from build123d import *

# Parameters (mm, degrees)
EXTRUDE_1_DEPTH     = 5
EXTRUDE_1_2_DEPTH   = 5
EXTRUDE_1_3_DEPTH   = 5
EXTRUDE_1_4_DEPTH   = 5
EXTRUDE_3_DEPTH     = 2
SKETCH_3_W          = 20
SKETCH_3_H          = 19.604409946
CUT_EXTRUDE_1_DEPTH = 2
SKETCH_4_R          = 1.5
CUT_EXTRUDE_2_DEPTH = 12
SKETCH_6_W          = 24.27884079
SKETCH_6_H          = 14.237664084
CUT_EXTRUDE_5_DEPTH = 10


with BuildPart() as part:
    # Sketch 1 → Extrude 1 (new body)
    with BuildSketch(Plane.XY):
        with BuildLine():
            Line((13.964240044, 24), (-13.964240044, 24))
            ThreePointArc((-13.964240044, 24), (0, 11), (13.964240044, 24))
        make_face()
    extrude(amount=-EXTRUDE_1_DEPTH)



with BuildPart() as body_2:
    # Sketch 1 → Extrude 1 2 (new body)
    with BuildSketch(Plane.XY):
        with BuildLine():
            ThreePointArc((-18, -12.124355653), (-11, 0), (-18, 12.124355653))
            Line((-18, 12.124355653), (-18, -12.124355653))
        make_face()
    extrude(amount=-EXTRUDE_1_2_DEPTH)


with BuildPart() as body_3:
    # Sketch 1 → Extrude 1 3 (new body)
    with BuildSketch(Plane.XY):
        with BuildLine():
            Line((18, -12.124355653), (18, 12.124355653))
            ThreePointArc((18, 12.124355653), (11, 0), (18, -12.124355653))
        make_face()
    extrude(amount=-EXTRUDE_1_3_DEPTH)


with BuildPart() as body_4:
    # Sketch 1 → Extrude 1 4 (new body)
    with BuildSketch(Plane.XY):
        with BuildLine():
            ThreePointArc((13.964240044, -24), (0, -11), (-13.964240044, -24))
            Line((-13.964240044, -24), (13.964240044, -24))
        make_face()
    extrude(amount=-EXTRUDE_1_4_DEPTH)


with BuildPart() as part_1:
    add(part.part)

    add(body_2.part)  # Extrude 3 merges body 2

    add(body_3.part)  # Extrude 3 merges body 3

    add(body_4.part)  # Extrude 3 merges body 4
    # Sketch 2 → Extrude 3 (add)
    with BuildSketch(Plane.XY):
        with BuildLine():
            ThreePointArc((-18, 22.45), (-19.096015511, 25.096015511), (-16.45, 24))
            Line((-16.45, 24), (-12.139420395, 24))
            ThreePointArc((-12.139420395, 24), (-22.14405558, 28.14405558), (-18, 18.139420395))
            Line((-18, 18.139420395), (-18, 22.45))
        make_face()
        with BuildLine():
            Line((-12.139420395, 24), (-16.45, 24))
            ThreePointArc((-16.45, 24), (-16.903984489, 22.903984489), (-18, 22.45))
            Line((-18, 22.45), (-18, 18.139420395))
            ThreePointArc((-18, 18.139420395), (-13.85594442, 19.85594442), (-12.139420395, 24))
        make_face()
        with BuildLine():
            Line((12.139420395, 24), (-12.139420395, 24))
            ThreePointArc((-12.139420395, 24), (-13.85594442, 19.85594442), (-18, 18.139420395))
            Line((-18, 18.139420395), (-18, 12.124355653))
            ThreePointArc((-18, 12.124355653), (-11, 0), (-18, -12.124355653))
            Line((-18, -12.124355653), (-18, -18.139420395))
            ThreePointArc((-18, -18.139420395), (-13.85594442, -19.85594442), (-12.139420395, -24))
            Line((-12.139420395, -24), (12.139420395, -24))
            ThreePointArc((12.139420395, -24), (13.85594442, -19.85594442), (18, -18.139420395))
            Line((18, -18.139420395), (18, 18.139420395))
            ThreePointArc((18, 18.139420395), (13.85594442, 19.85594442), (12.139420395, 24))
        make_face()
        with BuildLine():
            ThreePointArc((-18, -12.124355653), (-11, 0), (-18, 12.124355653))
            Line((-18, 12.124355653), (-18, -12.124355653))
        make_face()
        with BuildLine():
            ThreePointArc((23.860579605, 24), (18, 29.860579605), (12.139420395, 24))
            Line((12.139420395, 24), (16.45, 24))
            ThreePointArc((16.45, 24), (18, 25.55), (19.55, 24))
            ThreePointArc((19.55, 24), (19.096015511, 22.903984489), (18, 22.45))
            Line((18, 22.45), (18, 18.139420395))
            ThreePointArc((18, 18.139420395), (22.14405558, 19.85594442), (23.860579605, 24))
        make_face()
        with BuildLine():
            Line((16.45, 24), (12.139420395, 24))
            ThreePointArc((12.139420395, 24), (13.85594442, 19.85594442), (18, 18.139420395))
            Line((18, 18.139420395), (18, 22.45))
            ThreePointArc((18, 22.45), (16.903984489, 22.903984489), (16.45, 24))
        make_face()
        with BuildLine():
            ThreePointArc((-12.139420395, -24), (-13.85594442, -19.85594442), (-18, -18.139420395))
            Line((-18, -18.139420395), (-18, -22.45))
            ThreePointArc((-18, -22.45), (-16.903984489, -22.903984489), (-16.45, -24))
            Line((-16.45, -24), (-12.139420395, -24))
        make_face()
        with BuildLine():
            Line((-18, -22.45), (-18, -18.139420395))
            ThreePointArc((-18, -18.139420395), (-22.14405558, -28.14405558), (-12.139420395, -24))
            Line((-12.139420395, -24), (-16.45, -24))
            ThreePointArc((-16.45, -24), (-19.096015511, -25.096015511), (-18, -22.45))
        make_face()
        with BuildLine():
            ThreePointArc((23.860579605, -24), (22.14405558, -19.85594442), (18, -18.139420395))
            Line((18, -18.139420395), (18, -22.45))
            ThreePointArc((18, -22.45), (19.096015511, -22.903984489), (19.55, -24))
            ThreePointArc((19.55, -24), (18, -25.55), (16.45, -24))
            Line((16.45, -24), (12.139420395, -24))
            ThreePointArc((12.139420395, -24), (18, -29.860579605), (23.860579605, -24))
        make_face()
        with BuildLine():
            Line((18, -22.45), (18, -18.139420395))
            ThreePointArc((18, -18.139420395), (13.85594442, -19.85594442), (12.139420395, -24))
            Line((12.139420395, -24), (16.45, -24))
            ThreePointArc((16.45, -24), (16.903984489, -22.903984489), (18, -22.45))
        make_face()
    extrude(amount=EXTRUDE_3_DEPTH)

    # Sketch 3 → Cut-Extrude 1 (cut)
    with BuildSketch(Plane(origin=(0, 0, 0), x_dir=(-1, 0, 0), z_dir=(0, 0, -1))):
        Rectangle(SKETCH_3_W, SKETCH_3_H)
    extrude(amount=-CUT_EXTRUDE_1_DEPTH, mode=Mode.SUBTRACT)

    # Sketch 4 → Cut-Extrude 2 (cut)
    with BuildSketch(Plane(origin=(0, 0, -5), x_dir=(-1, 0, 0), z_dir=(0, 0, -1))):
        with Locations((21.25, -21.25)):
            Circle(SKETCH_4_R)
        with Locations((21.25, 21.25)):
            Circle(SKETCH_4_R)
        with Locations((-21.25, 21.25)):
            Circle(SKETCH_4_R)
        with Locations((-21.25, -21.25)):
            Circle(SKETCH_4_R)
    extrude(amount=-CUT_EXTRUDE_2_DEPTH, mode=Mode.SUBTRACT)

    # Sketch 6 → Cut-Extrude 5 (cut)
    with BuildSketch(Plane.XY.offset(2)):
        with Locations((0, -24)):
            Rectangle(SKETCH_6_W, SKETCH_6_H)
    extrude(amount=-CUT_EXTRUDE_5_DEPTH, mode=Mode.SUBTRACT)


solid = part_1.part
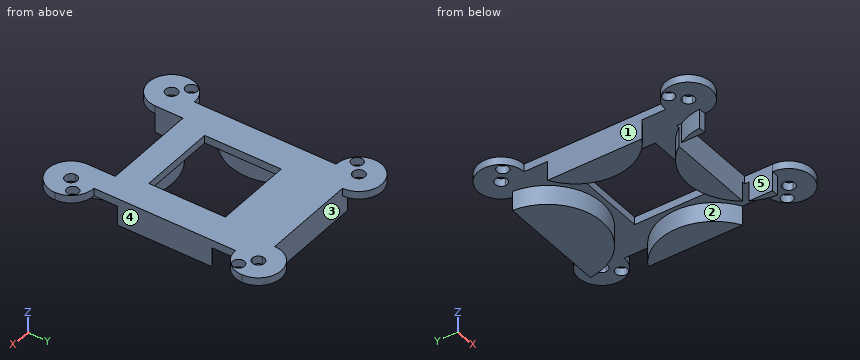
Here's how the part is built. I have some questions about the finished solid (model axes, mm). Face numbers are marked on the shaded views. A direction names the side the tool comes from. Round coordinates to 2 decimals unless told otherwise and drop trailing zeros. Write each loop counter-clockwise with the first axis right and the second up, starting at its lowest first coordinate (ties: lowest second). Pieces come first, ordered by that corner, then holes.
1. Will these pins go through, and if not, where does the flat tip stop? pin 1 Ø3.5 at (x, y) = (-18, 24) entering from -Z; pin 2 Ø3 at (x, y) = (-18, -24) entering from +Z; pin 3 Ø1.6 at (y, z) = (-0.5, 1) entering from +X; pin 4 Ø1 at (y, z) = (22.5, 0) entering from +X.
2. Suppose I cut it at C-C (y = 21.25). List the corners of the cut face in (x, z) for me.
3. Suppose I cut it at A-A (z = -0.75). List the corners of the cut face in (x, y) for me, and give its area (3 significant figures).
4. For the marked faces 1, 2, 3, 4 and 5, which set-ups out of +Z, -Z, +X, -X, +Y, -Y let a thin tool reach every point of the face, with its end or its side?
5. Suppose I cut it at D-D (y = -21.25). List the corners of the cut face in (x, z) for me.
6. Suppose I cut it at B-B (x = 7). List the corners of the cut face in (y, z) for me, and give its area (3 significant figures).
7. I need wall thicknesses on L1, parallel to X at y = -24, z = 0.7; L2, parallel to Y at x = -21.25, z = 0.45; L3, parallel to Y at x = 7, z = 0.5. Which ranges of each line are inside material? Lowest first, please.
Answer sheet:
1. pin 1: stops at z = 0
1. pin 2: passes through
1. pin 3: stops at x = 18
1. pin 4: stops at x = 23.77
2. outline: (-23.18, 0) - (-22.75, 0) - (-22.75, 2) - (-23.18, 2) - close; (-19.75, 0) - (-13.49, 0) - (-13.49, -5) - (13.49, -5) - (13.49, 0) - (19.75, 0) - (19.75, 2) - (-19.75, 2) - close; (22.75, 0) - (23.18, 0) - (23.18, 2) - (22.75, 2) - close
3. outline: (-18, -12.12) arc R14 ccw to (-18, 12.12) - close; (-13.96, -24) - (-12.14, -24) - (-12.14, -18.03) arc R14 ccw to start; (-13.96, 24) arc R14 ccw to (13.96, 24) - close; (-11.41, -16.88) - (11.41, -16.88) arc R14 ccw to start; (12.14, -24) - (13.96, -24) arc R14 ccw to (12.14, -18.03) - close; (18, -12.12) - (18, 12.12) arc R14 ccw to start
3. area: 629 mm2
4. face 1: +Z, -Z, -X
4. face 2: -Z
4. face 3: -Z, +Y
4. face 4: +Z, -Z, +X
4. face 5: +Z, -Z, -Y
5. outline: (-23.18, 0) - (-22.75, 0) - (-22.75, 2) - (-23.18, 2) - close; (-19.75, 0) - (-13.49, 0) - (-13.49, -5) - (-12.14, -5) - (-12.14, 2) - (-19.75, 2) - close; (12.14, -5) - (13.49, -5) - (13.49, 0) - (19.75, 0) - (19.75, 2) - (12.14, 2) - close; (22.75, 0) - (23.18, 0) - (23.18, 2) - (22.75, 2) - close
6. outline: (-16.88, -5) - (-12.88, -5) - (-12.88, 0) - (-9.8, 0) - (-9.8, 2) - (-16.88, 2) - close; (9.8, 0) - (12.88, 0) - (12.88, -5) - (24, -5) - (24, 2) - (9.8, 2) - close
6. area: 118 mm2
7. L1: x = -23.86 to -19.55, -16.45 to -12.14, 12.14 to 16.45, 19.55 to 23.86
7. L2: y = -28.88 to -22.75, -19.75 to -19.12, 19.12 to 19.75, 22.75 to 28.88
7. L3: y = -16.88 to -9.8, 9.8 to 24
